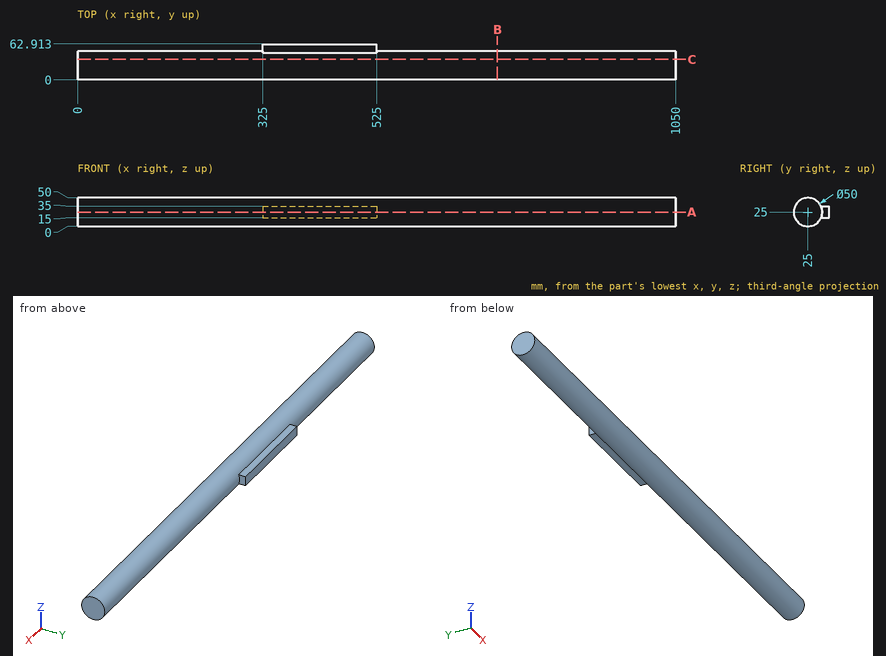
Design review of the part shown in the three views and the two pictorial views. Dimensions are in mm from the part's minimum x, y and z. Round coordinates to 2 decimals unless told otherwise and drop trailing zeros. Loops run counter-clockwise (first coordinate to the right, second up) from the corner with the lowest first, then second, coordinate; pieces in that order, holes last. Notation, with made-up numbers: M -30,26 L 14,26 A10 ccw 14,41 Z; hole C 79.25,11 d7. An arc over 180 degrees is marked long. Answer as a JSON object with one key per item and string values.
Item 1: For line 1 along Z through (x, y) = (842.5, 23.5) (3 decimals); line 2 along Z through (x, y) = (129.5, 48); line 3 along X through (y, z) = (60.5, 24), list the stretches that pass through material, from the lowest coordinate up.
Check sheet entries:
{"line 1": "0.045 to 49.955", "line 2": "15.2 to 34.8", "line 3": "325 to 525"}
Item 2: We need section C-C, the plane y = 36. State the section outline as (x, z) points.
Check sheet entries:
{"outline": "M 0,2.55 L 1050,2.55 L 1050,47.45 L 0,47.45 Z"}
Item 3: Clearance check with flat-ended pins moving along their axes: P1, Ø8, axis at x = 262, y = 56, coming from the +Z side; P2, Ø1, axis at x = 253.5, y = 22, coming from the +Z side; P3, Ø12, axis at x = 898.5, y = 11, coming from the +Z side; P4, Ø3, axis at x = 219.5, z = 42, coming from the +Y side (3 decimals). State where each tip first meets the part, or that it passes through.
Check sheet entries:
{"P1": "through", "P2": "z = 49.87", "P3": "z = 48.69", "P4": "y = 44.615"}
Item 4: We need section A-A, the plane z = 25. State the section outline as (x, y) points.
Check sheet entries:
{"outline": "M 0,0 L 1050,0 L 1050,50 L 525,50 L 525,62.91 L 325,62.91 L 325,50 L 0,50 Z"}
Item 5: We need section B-B, the plane x = 737. State the section outline as (y, z) points.
Check sheet entries:
{"outline": "C 25,25 d50"}
